Work out the finished part from the listing and answer in its coordinate system (mm). Face numbers are marked on the shaded views. A direction names the side the tool comes from. Round coordinates to 2 decimals unless told otherwise and drop trailing zeros. Loops run counter-clockwise (first coordinate to the right, second up) from the corner with the lowest first, then second, coordinate; pieces in that order, holes last. Notation, with made-up numbers: (16.25, -13) - (35.25, -13) arc R23 ccw to (35.25, 6) - close; hole circle Ø4 at (56.5, 84). An arc over 180 degrees is marked (long way). Answer as CSV lines item,"result". Start each with the question number.
Q1. Section A-A on x = 6.5 is taken. Write down the section's boundary in (y, z), then the cut area to 3 significant figures.
Q2. Section B-B on y = -8.5 is taken. Write down the section's boundary in (x, z), then the cut area to 3 significant figures.
Q3. Each of these flat-tipped pins is pushed along its axis until it touches: pin 1 Ø8 at (x, z) = (-10.5, -3) entering from -Y; pin 2 Ø1.5 at (x, y) = (6.5, 1.5) entering from -Z; pin 3 Ø8 at (x, z) = (-5, -10.5) entering from +Y; pin 4 Ø7 at (x, y) = (-2, 3.5) entering from -Z. Where does it stop, or does it pass through?
Q4. Straight lines are drawn through the part: L1, parallel to X at y = 3, z = -10; L2, parallel to Z at x = 6, y = 2.5; L3, parallel to Z at x = 8.5, y = -13. For each, find the intervals that lie inside material, in ascending order. Write a range as [from, to].
Q5. For the marked faces 1 and 2, determine the directions among +Z, -Z, +X, -X, +Y, -Y from which every point of the face is accessible in a straight line to the end or side of a thin tool.
Q6. Section C-C on z = -11.5 is taken. Write down the section's boundary in (x, y), then the cut area to 3 significant figures.
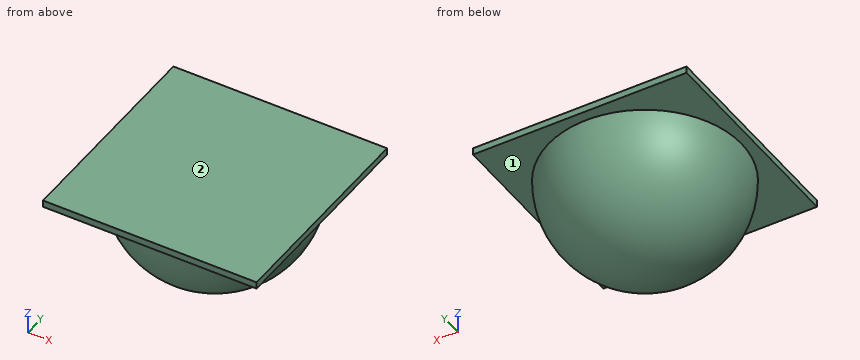
```python
from build123d import *

# Parameters (mm, degrees)
SHELL1_T            = -2
SKETCH3_W           = 31
SKETCH3_H           = 31
BOSS_EXTRUDE1_DEPTH = 1


with BuildPart() as part:
    # Sketch1 → Revolve1 (revolve)
    with BuildSketch(Plane(origin=(0, 0, 0), x_dir=(1, 0, 0), z_dir=(0, 1, 0))):
        with BuildLine():
            Line((0, 14), (0, 0))
            Line((0, 0), (14, 0))
            ThreePointArc((14, 0), (9.899494937, 9.899494937), (0, 14))
        make_face()
    revolve(axis=Axis((0, 0, -14), (0, 0, 1)))

    # Shell1
    shell1_openings = [part.faces().sort_by_distance(p)[0] for p in [
        (0, 0, 0),
    ]]
    offset(amount=SHELL1_T, openings=shell1_openings, kind=Kind.INTERSECTION)

    # Sketch3 → Boss-Extrude1 (add)
    with BuildSketch(Plane.XY):
        Rectangle(SKETCH3_W, SKETCH3_H)
    extrude(amount=BOSS_EXTRUDE1_DEPTH)


solid = part.part
```
Findings:
1,outline,"(-15.5, 0) - (-12.4, 0) arc R12.4 ccw to (12.4, 0) - (15.5, 0) - (15.5, 1) - (-15.5, 1) - close; hole (-10.09, 0) arc R10.09 ccw to (10.09, 0) - close"
1,area,"113 mm^2"
2,outline,"(-15.5, 0) - (-11.12, 0) arc R11.12 ccw to (11.12, 0) - (15.5, 0) - (15.5, 1) - (-15.5, 1) - close; hole (-8.47, 0) arc R8.47 ccw to (8.47, 0) - close"
2,area,"113 mm^2"
3,pin 1,"stops at y = -15.5"
3,pin 2,"stops at z = -12.69"
3,pin 3,"stops at y = 11.74"
3,pin 4,"stops at z = -13.99"
4,L1,"x = [-9.33, -5.92], [5.92, 9.33]"
4,L2,"z = [-12.4, -10.09], [0, 1]"
4,L3,"z = [0, 1]"
5,face 1,"-Z"
5,face 2,"+Z, +X, -X, +Y, -Y"
6,outline,"circle Ø15.97 at (0, 0); hole circle Ø6.86 at (0, 0)"
6,area,"163 mm^2"
